Design review of the part built by this model. Coordinates are the model's own, in mm. Face numbers are marked on the shaded views. Give positions to 0.01 mm unless a question says otherwise; leave off trailing zeros. Write each loop counter-clockwise with the first axis right and the second up, starting at its lowest first coordinate (ties: lowest second). Pieces come first, ordered by that corner, then holes. Notation, with made-up numbers: M 67,17 L 91,17 A7 ccw 91,26 Z; hole C -30.5,-24.5 d2. An arc over 180 degrees is marked long. Write each question's results on one line, items separated by ' | '. Start each with the question number.
from build123d import *

# Parameters (mm, degrees)
EXTRUDE_1_DEPTH     = 8
SKETCH_2_R          = 3.2
CUT_EXTRUDE_1_DEPTH = 2
SKETCH_3_W          = 40
SKETCH_3_H          = 30
EXTRUDE_2_DEPTH     = 2
EXTRUDE_3_DEPTH     = 16
FILLET_1_R          = 2
SKETCH_4_R          = 1.6
CUT_EXTRUDE_3_DEPTH = 51.042481953


with BuildPart() as part:
    # Sketch 1 → Extrude 1 (new body)
    with BuildSketch(Plane.XY):
        with BuildLine():
            ThreePointArc((-11.6, 5), (-10, 6.6), (-8.4, 5))
            Line((-8.4, 5), (-7.5, 5))
            Line((-7.5, 5), (-7.5, 9.330127019))
            ThreePointArc((-7.5, 9.330127019), (-10, 10), (-12.5, 9.330127019))
            Line((-12.5, 9.330127019), (-12.5, 5))
            Line((-12.5, 5), (-11.6, 5))
        make_face()
        with BuildLine():
            Line((-7.5, 5), (-8.4, 5))
            ThreePointArc((-8.4, 5), (-10, 3.4), (-11.6, 5))
            Line((-11.6, 5), (-12.5, 5))
            Line((-12.5, 5), (-12.5, 9.330127019))
            ThreePointArc((-12.5, 9.330127019), (-12.5, 0.669872981), (-5, 5))
            ThreePointArc((-5, 5), (-5.669872981, 7.5), (-7.5, 9.330127019))
            Line((-7.5, 9.330127019), (-7.5, 5))
        make_face()
        with BuildLine():
            ThreePointArc((-12.5, 9.330127019), (-10, 10), (-7.5, 9.330127019))
            Line((-7.5, 9.330127019), (-7.5, 13))
            Line((-7.5, 13), (-12.5, 13))
            Line((-12.5, 13), (-12.5, 9.330127019))
        make_face()
    extrude(amount=-EXTRUDE_1_DEPTH)

    # Sketch 2 → Cut-Extrude 1 (cut)
    with BuildSketch(Plane.XY):
        with Locations((-10, 5)):
            Circle(SKETCH_2_R)
    extrude(amount=-CUT_EXTRUDE_1_DEPTH, mode=Mode.SUBTRACT)

    # Sketch 3 → Extrude 2 (add)
    with BuildSketch(Plane(origin=(0, 13, 0), x_dir=(1, 0, 0), z_dir=(0, 1, 0))):
        with Locations((-22.5, 8)):
            Rectangle(SKETCH_3_W, SKETCH_3_H)
    extrude(amount=EXTRUDE_2_DEPTH)

    # Sketch 1_3 → Extrude 3 (add)
    with BuildSketch(Plane.XY):
        with BuildLine():
            ThreePointArc((-12.5, 9.330127019), (-10, 10), (-7.5, 9.330127019))
            Line((-7.5, 9.330127019), (-7.5, 13))
            Line((-7.5, 13), (-12.5, 13))
            Line((-12.5, 13), (-12.5, 9.330127019))
        make_face()
    extrude(amount=-EXTRUDE_3_DEPTH)

    # Fillet 1
    fillet_1_edges = [part.edges().sort_by_distance(p)[0] for p in [
        (-42.5, 14, -23),
        (-42.5, 14, 7),
        (-2.5, 14, 7),
        (-2.5, 14, -23),
    ]]
    fillet(fillet_1_edges, radius=FILLET_1_R)

    # Sketch 4 → Cut-Extrude 3 (cut, through all)
    with BuildSketch(Plane.XZ.offset(-13)):
        with Locations((-5.5, 4)):
            Circle(SKETCH_4_R)
        with Locations((-5.5, -20)):
            Circle(SKETCH_4_R)
        with Locations((-39.5, -20)):
            Circle(SKETCH_4_R)
        with Locations((-39.5, 4)):
            Circle(SKETCH_4_R)
    extrude(amount=-CUT_EXTRUDE_3_DEPTH, mode=Mode.SUBTRACT)


solid = part.part
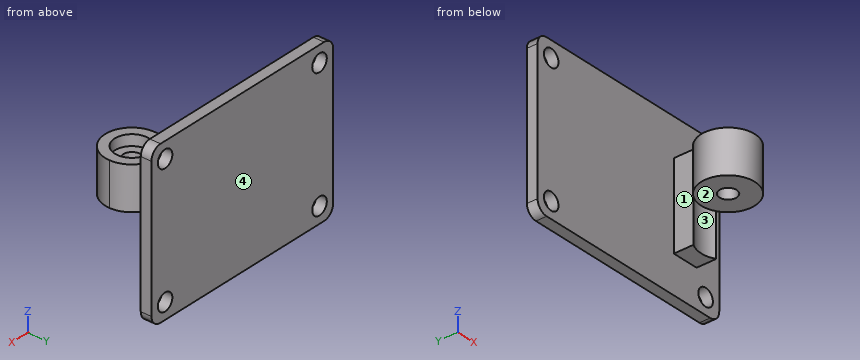
Q1. We need section A-A on z = -20. Write out the cut boundary in (x, y), and give its area (3 significant figures).
Q2. We need section B-B on x = -10. Write out the cut boundary in (y, z), and give its area (3 significant figures).
Q3. The part is to be moulded in two halves that separate along Y. For the marked faces 1, 2, 3 and 4, say which applies: pulls with the +Y half, pulls with the -Y half, needs draft (parallel to the pull), parting line crosses it, or undercut.
Q4. Wall thickness on line 1 along Z through (x, y) = (-5.5, 13.8); line 2 along Y through (x, z) = (-10, -4.3); line 3 along Y through (x, z) = (-23.5, 2.25): over which ranges is each line inside the solid? List them lowest first. Write a range as from..to.
Q5. We need section D-D on z = -12.25. Write out the cut boundary in (x, y), and give its area (3 significant figures).
Q6. For pin 1 Ø4 at (x, y) = (-10, 5) entering from +Z; pin 2 Ø3 at (x, y) = (-11, 10.5) entering from -Z; pin 3 Ø1.1 at (y, z) = (10.5, -11) entering from -X, all flat-tipped, find the tip position at first contact; note any pin that passes through.
Q7. We need section C-C on x = -39.5. Write out the cut boundary in (y, z), and give its area (3 significant figures).
Answer sheet:
1) outline: M -42.5,13 L -41.1,13 L -41.1,15 L -42.5,15 Z; M -37.9,13 L -7.1,13 L -7.1,15 L -37.9,15 Z; M -3.9,13 L -2.5,13 L -2.5,15 L -3.9,15 Z | area: 67.2 mm^2
2) outline: M 0,-8 L 3.4,-8 L 3.4,-2 L 1.8,-2 L 1.8,0 L 0,0 Z; M 6.6,-8 L 10,-8 L 10,-16 L 13,-16 L 13,-23 L 15,-23 L 15,7 L 13,7 L 13,0 L 8.2,0 L 8.2,-2 L 6.6,-2 Z | area: 156 mm^2
3) face 1: undercut | face 2: needs draft | face 3: pulls with the -Y half | face 4: pulls with the +Y half
4) line 1: -23..-21.6, -18.4..2.4, 5.6..7 | line 2: 0..3.4, 6.6..15 | line 3: 13..15
5) outline: M -42.5,13 L -12.5,13 L -12.5,9.33 A5 cw -7.5,9.33 L -7.5,13 L -2.5,13 L -2.5,15 L -42.5,15 Z | area: 96.1 mm^2
6) pin 1: z = -2 | pin 2: z = -16 | pin 3: x = -12.5
7) outline: M 13,-23 L 15,-23 L 15,-21.6 L 13,-21.6 Z; M 13,-18.4 L 15,-18.4 L 15,2.4 L 13,2.4 Z; M 13,5.6 L 15,5.6 L 15,7 L 13,7 Z | area: 47.2 mm^2
